Geometry: final body of the model. Coordinates: model frame, mm. Coordinates: 2 decimals unless noted, no trailing zeros. Order: outer loops, then holes, each group sorted by start corner. A loop starts at its lowest first (then second) coordinate and runs counter-clockwise, first axis right, second up. Notation, with made-up numbers: (-40, -19) -> (11, -19) arc R31 ccw to (11, 20) -> close; hole circle Ø5 at (0, 75.5). An arc over 180 degrees is marked (long way). Answer in a Markdown table with one row per item. Add a question column.
1) Section query C-C on y = -14. Return the cut outline in (x, z).
2) Section query B-B on z = 0.4. Return the cut outline in (x, y), then the cut area to 3 significant figures.
3) Section query A-A on x = 0. Return the cut outline in (y, z).
4) Ray query, line 1 (Y direction, x = 0, z = 1.6); line 2 (Y direction, x = 15.5, z = 1.7); line 3 (X direction, y = 3.5, z = 0.6). Return the intervals inside material, ascending. Write a range as from..to.
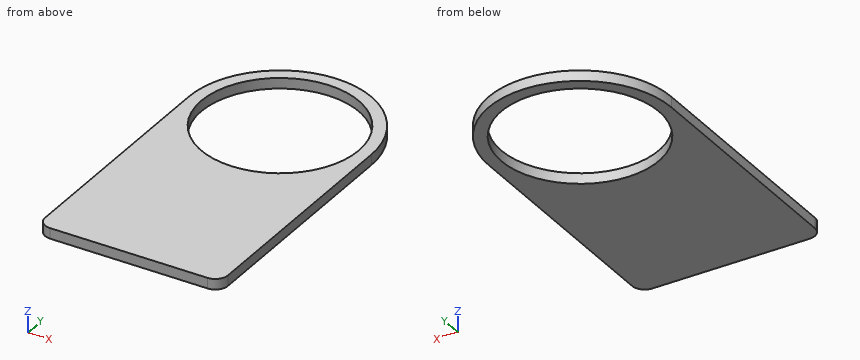
```python
from build123d import *

# Parameters (mm, degrees)
SKETCH_R  = 18.75
PAD_DEPTH = 2.5
FILLET_R  = 3


with BuildPart() as part:
    # Sketch → Pad (new body)
    with BuildSketch(Plane.XY):
        with BuildLine():
            Line((21.75, 0), (21.75, -58.75))
            Line((21.75, -58.75), (-21.75, -58.75))
            Line((-21.75, -58.75), (-21.75, 0))
            ThreePointArc((21.75, 0), (0, 21.75), (-21.75, 0))
        make_face()
        Circle(SKETCH_R, mode=Mode.SUBTRACT)
    extrude(amount=PAD_DEPTH)

    # Fillet
    fillet_edges = [part.edges().sort_by_distance(p)[0] for p in [
        (-21.75, -58.75, 1.25),
        (21.75, -58.75, 1.25),
    ]]
    fillet(fillet_edges, radius=FILLET_R)


solid = part.part
```
Result:
| question | item | result |
|---|---|---|
| 1 | outline | (-21.75, 0) -> (-12.47, 0) -> (-12.47, 2.5) -> (-21.75, 2.5) -> close; (12.47, 0) -> (21.75, 0) -> (21.75, 2.5) -> (12.47, 2.5) -> close |
| 2 | outline | (-21.75, -55.75) arc R3 ccw to (-18.75, -58.75) -> (18.75, -58.75) arc R3 ccw to (21.75, -55.75) -> (21.75, 0) arc R21.75 ccw to (-21.75, 0) -> close; hole circle Ø37.5 at (0, 0) |
| 2 | area | 2,190 mm2 |
| 3 | outline | (-58.75, 0) -> (-18.75, 0) -> (-18.75, 2.5) -> (-58.75, 2.5) -> close; (18.75, 0) -> (21.75, 0) -> (21.75, 2.5) -> (18.75, 2.5) -> close |
| 4 | line 1 | -58.75..-18.75, 18.75..21.75 |
| 4 | line 2 | -58.75..-10.55, 10.55..15.26 |
| 4 | line 3 | -21.47..-18.42, 18.42..21.47 |
